The model under review builds one solid part; all positions refer to its coordinate system, in mm. A direction names the side the tool comes from. Coordinates: 2 decimals unless noted, no trailing zeros. Order: outer loops, then holes, each group sorted by start corner. A loop starts at its lowest first (then second) coordinate and runs counter-clockwise, first axis right, second up. Notation, with made-up numbers: (71, 7.5) -> (75, 7.5) arc R24 cw to (75, 41.5) -> close; hole circle Ø4 at (-0.75, -5.75). An arc over 180 degrees is marked (long way). Use one line per item in the form item = value. Start each with the question number.
(1) Take a section at A-A (z = 4.5). State the section outline as (x, y) points, then the cut area to 4 significant figures.
(2) Take a section at D-D (z = -3.75). State the section outline as (x, y) points.
(3) Take a section at C-C (x = 8.5). State the section outline as (y, z) points.
(4) Mouldability with a two-part tool opening along Y and no side actions: class faces 1 (the flat face through (-14, 17.5, 0)), 2 (the flat face through (5, 28, 0)), 3 (the flat face through (0, 12, 6)) as +Y half, -Y half, draft (parallel to the pull), parting line (faces both ways), or undercut.
(5) For faces 4 (the flat face through (-11.5, 22, 0)), 5 (the cylindrical face through (0.74, 25.97, 3.65)), 6 (the flat face through (14, 20, 0)), 7 (the flat face through (11.5, 9, 0)), 8 (the flat face through (10, 24, -5)), list the 3-axis set-ups (+Z, -Z, +X, -X, +Y, -Y) from which the entire face can be reached by the end or side of a thin tool; tool diameter is ignored.
(6) Insertion check: pin 1 Ø1.5 at (y, z) = (24, 3.5) entering from -X; pin 2 Ø4 at (x, z) = (-3, 1.5) entering from +Y; pin 3 Ø1.4 at (x, z) = (14, -3) entering from +Y. Each pin has a flat end and moves straight along its axis. Give the tip position at first contact, or say it passes through.
(7) Take a section at B-B (y = 7.75). State the section outline as (x, z) points, then the cut area to 3 significant figures.
(8) Wall thickness on line 1 along X through (y, z) = (10.25, 3); line 2 along Y through (x, z) = (13, 3.5); line 3 along Y through (x, z) = (-2, -2): over which ranges is each line inside the solid? List them lowest first.
```python
from build123d import *

# Parameters (mm, degrees)
SKETCH1_R           = 6
BOSS_EXTRUDE1_DEPTH = 24
BOSS_EXTRUDE2_START = 24
SKETCH1_3_R         = 6
BOSS_EXTRUDE2_DEPTH = 4
BOSS_EXTRUDE3_START = 20
SKETCH1_4_W         = 32.5
SKETCH1_4_H         = 12
BOSS_EXTRUDE3_DEPTH = 2.5


with BuildPart() as part:
    # Sketch1 → Boss-Extrude1 (new body)
    with BuildSketch(Plane(origin=(0, 0, 0), x_dir=(1, 0, 0), z_dir=(0, 1, 0))):
        with BuildLine():
            Line((-11.5, 6), (-11.5, -6))
            Line((-11.5, -6), (5.5, -6))
            ThreePointArc((5.5, -6), (-0.5, -3e-09), (5.499999994, 6))
            Line((5.499999994, 6), (-11.5, 6))
        make_face()
        with Locations((5.5, 0)):
            Circle(SKETCH1_R)
        with BuildLine():
            Line((11.5, 6), (5.499999994, 6))
            ThreePointArc((5.499999994, 6), (9.742640685, 4.242640689), (11.5, 0))
            Line((11.5, 0), (11.5, 6))
        make_face()
        with BuildLine():
            ThreePointArc((11.5, 0), (9.742640687, -4.242640687), (5.5, -6))
            Line((5.5, -6), (11.5, -6))
            Line((11.5, -6), (11.5, 0))
        make_face()
    extrude(amount=BOSS_EXTRUDE1_DEPTH)

    # Sketch1<3> → Boss-Extrude2 (add)
    with BuildSketch(Plane(origin=(0, 0, 0), x_dir=(1, 0, 0), z_dir=(0, 1, 0)).offset(BOSS_EXTRUDE2_START)):
        with Locations((5.5, 0)):
            Circle(SKETCH1_3_R)
    extrude(amount=BOSS_EXTRUDE2_DEPTH)

    # Sketch1<4> → Boss-Extrude3 (add)
    with BuildSketch(Plane(origin=(0, 0, 0), x_dir=(1, 0, 0), z_dir=(0, 1, 0)).offset(BOSS_EXTRUDE3_START)):
        Rectangle(SKETCH1_4_W, SKETCH1_4_H)
    extrude(amount=-BOSS_EXTRUDE3_DEPTH)


solid = part.part
```
Findings:
q1.outline = (-16.25, 17.5) -> (-11.5, 17.5) -> (-11.5, 0) -> (11.5, 0) -> (11.5, 17.5) -> (16.25, 17.5) -> (16.25, 20) -> (11.5, 20) -> (11.5, 24) -> (9.47, 24) -> (9.47, 28) -> (1.53, 28) -> (1.53, 24) -> (-11.5, 24) -> (-11.5, 20) -> (-16.25, 20) -> close
q1.area = 607.5 mm²
q2.outline = (-16.25, 17.5) -> (-11.5, 17.5) -> (-11.5, 0) -> (11.5, 0) -> (11.5, 17.5) -> (16.25, 17.5) -> (16.25, 20) -> (11.5, 20) -> (11.5, 24) -> (10.18, 24) -> (10.18, 28) -> (0.82, 28) -> (0.82, 24) -> (-11.5, 24) -> (-11.5, 20) -> (-16.25, 20) -> close
q3.outline = (0, -6) -> (24, -6) -> (24, -5.2) -> (28, -5.2) -> (28, 5.2) -> (24, 5.2) -> (24, 6) -> (0, 6) -> close
q4.face_1 = -Y half
q4.face_2 = +Y half
q4.face_3 = draft
q5.face_4 = +Z, -Z, -X, +Y
q5.face_5 = +Y
q5.face_6 = +Z, -Z, +X, +Y
q5.face_7 = +Z, -Z, +X, -Y
q5.face_8 = -Z, +X, +Y
q6.pin_1 = -11.5
q6.pin_2 = 24
q6.pin_3 = 20
q7.outline = (-11.5, -6) -> (11.5, -6) -> (11.5, 6) -> (-11.5, 6) -> close
q7.area = 276 mm²
q8.line_1 = -11.5 to 11.5
q8.line_2 = 17.5 to 20
q8.line_3 = 0 to 24
